Part model, mm, in its own coordinate system. Coordinates: 2 decimals unless noted, no trailing zeros. Order: outer loops, then holes, each group sorted by start corner. A loop starts at its lowest first (then second) coordinate and runs counter-clockwise, first axis right, second up.
from build123d import *

# Parameters (mm, degrees)
F0_W     = 40
F0_H     = 2
F1_DEPTH = 20
F4_D     = 8
F5_D     = 2


with BuildPart() as f1:
    # F0 (on Top) → F1 (new body)
    with BuildSketch(Plane.XY):
        with Locations((-38.553373, 16.042135)):
            Rectangle(F0_W, F0_H)
    extrude(amount=F1_DEPTH)

    # F4 (through all)
    with Locations(Plane.XZ):
        with Locations((-37.980106, 9.301319)):
            Hole(F4_D / 2)

    # F5 (through all)
    with Locations(Plane.XZ):
        with Locations((-55.724628, 9.301319), (-21.106074, 9.301319)):
            Hole(F5_D / 2)


solid = f1.part
Q1. Mould opens along Z. For faces 1 (the face through (-20.37, 16.06, 9.98)), 2 (the face through (-39, 16, 0)), 3 (the face through (-56.68, 16.06, 9.6)), 4 (the face through (-18.553, 16, 10)) say: pulls with the +Z half, pulls with the -Z half, needs draft (parallel to the pull), parting line crosses it, or undercut.
Results list:
face 1: undercut
face 2: pulls with the -Z half
face 3: undercut
face 4: needs draft
Q2. Cut at B-B on y = 15.45. Write the cut outline in (x, z).
Results list:
outline: (-58.55, 0) - (-18.55, 0) - (-18.55, 20) - (-58.55, 20) - close; hole circle Ø2 at (-55.72, 9.3); hole circle Ø8 at (-37.98, 9.3); hole circle Ø2 at (-21.11, 9.3)
Q3. Cut at A-A on z = 11. Write the cut outline in (x, y).
Results list:
outline: (-58.55, 15.04) - (-41.6, 15.04) - (-41.6, 17.04) - (-58.55, 17.04) - close; (-34.36, 15.04) - (-18.55, 15.04) - (-18.55, 17.04) - (-34.36, 17.04) - close
Q4. Cut at C-C on x = -36.5. Write the cut outline in (y, z), and give its area (3 significant figures).
Results list:
outline: (15.04, 0) - (17.04, 0) - (17.04, 5.59) - (15.04, 5.59) - close; (15.04, 13.02) - (17.04, 13.02) - (17.04, 20) - (15.04, 20) - close
area: 25.1 mm2
Q5. Wall check: line 1 along X through (y, z) = (16.45, 9.75); line 2 along Z through (x, y) = (-38, 15.75); line 3 along X through (y, z) = (16, 12.75). Give the ranges that are in metal, low to high.
Results list:
line 1: x = -58.55 to -56.62, -54.83 to -41.95, -34.01 to -22, -20.21 to -18.55
line 2: z = 0 to 5.3, 13.3 to 20
line 3: x = -58.55 to -40.01, -35.95 to -18.55
